Source: CAD feature listing. Evaluate the final solid. Frame: model axes, mm. A direction names the side the tool comes from. Give positions to 0.01 mm unless a question says otherwise; leave off trailing zeros. Write each loop counter-clockwise with the first axis right and the second up, starting at its lowest first coordinate (ties: lowest second). Pieces come first, ordered by that corner, then holes. Notation, with made-up numbers: (1, 37.25) -> (23, 37.25) arc R14 cw to (23, 58.25) -> close; hole circle Ø3 at (33, 89.5). An arc over 180 degrees is marked (long way). Answer as a JSON object with one key per item and string values. Group by question number.
Item 1: Section query B-B on x = 7. Return the cut outline in (y, z), plus the area to 3 significant figures.
Item 2: Section query A-A on z = 72.5. Return the cut outline in (x, y).
Item 3: First-contact query: pin 1 Ø6.5 at (x, z) = (-19.05, -31.75) entering from -Y; pin 2 Ø4 at (y, z) = (0, -241.3) entering from -X. Flat tips, straight axial feed; report the tip coordinate or a pass-through.
Item 4: Access query for faces 5 (the face through (0, -11.112, 4)), 6 (the face through (0, 12.7, 4)). Directions: +Z, -Z, +X, -X, +Y, -Y. A direction counts if a zero-diameter tool reaches every point of the face in a straight line with its end or side. Return the directions, or none.
Item 5: Pull-direction query (X, two-part tool) for faces 1 (the face through (-23.812, 0, 4)), 2 (the face through (-25.4, 0, 4)), 3 (the face through (0, -12.7, 4)), 4 (the face through (25.4, 0, 4)); classes: pulls with the +X half, pulls with the -X half, needs draft (parallel to the pull), parting line crosses it, or undercut.
Item 6: Ray query, probe 1 along X at (y, z) = (12.35, -31.75); probe 2 along Z at (x, y) = (-19.05, 11.5); probe 3 along X at (y, z) = (-5, 212.5). Return the intervals inside material, ascending. Write a range as from..to.
from build123d import *

# Parameters (mm, degrees)
SKETCH1_W               = 50.8
SKETCH1_H               = 25.4
BOSS_EXTRUDE1_DEPTH     = 279.4
SHELL1_T                = -1.5875
CUT_EXTRUDE1_DEPTH      = 281.839473721
CUT_EXTRUDE1_DEPTH_BACK = 281.839473721
SKETCH3_R               = 2.4892
CUT_EXTRUDE2_DEPTH      = 281.839473721
CUT_EXTRUDE2_DEPTH_BACK = 281.839473721
SKETCH4_R               = 2.4892


with BuildPart() as part:
    # Sketch1 → Boss-Extrude1 (new, symmetric)
    with BuildSketch(Plane.XY):
        Rectangle(SKETCH1_W, SKETCH1_H)
    extrude(amount=BOSS_EXTRUDE1_DEPTH, both=True)

    # Shell1
    shell1_openings = [part.faces().sort_by_distance(p)[0] for p in [
        (0, 0, 279.4),
        (0, 0, -279.4),
    ]]
    offset(amount=SHELL1_T, openings=shell1_openings, kind=Kind.INTERSECTION)

    # Sketch3 → Cut-Extrude1 (cut, two sides: drawn at the far end of the back side and taken through both)
    with BuildSketch(Plane(origin=(0, 0, 0), x_dir=(0, 0, -1), z_dir=(1, 0, 0)).offset(-CUT_EXTRUDE1_DEPTH_BACK)):
        with Locations((-266.7, 0)):
            Circle(SKETCH3_R)
        with Locations((-241.3, 0)):
            Circle(SKETCH3_R)
        with Locations((-215.9, 0)):
            Circle(SKETCH3_R)
        with Locations((215.9, 0)):
            Circle(SKETCH3_R)
        with Locations((241.3, 0)):
            Circle(SKETCH3_R)
        with Locations((266.7, 0)):
            Circle(SKETCH3_R)
    extrude(amount=CUT_EXTRUDE1_DEPTH + CUT_EXTRUDE1_DEPTH_BACK, mode=Mode.SUBTRACT)

    # Sketch4 → Cut-Extrude2 (cut, two sides: drawn at the far end of the back side and taken through both)
    with BuildSketch(Plane(origin=(0, 0, 0), x_dir=(1, 0, 0), z_dir=(0, 1, 0)).offset(-CUT_EXTRUDE2_DEPTH_BACK)):
        with Locations(Location((0, -31.75, 0), (0, 0, 270))):
            Circle(SKETCH4_R)
        with Locations(Location((-19.05, -31.75, 0), (0, 0, 270))):
            Circle(SKETCH4_R)
        with Locations(Location((0, 31.75, 0), (0, 0, 270))):
            Circle(SKETCH4_R)
        with Locations(Location((-19.05, 31.75, 0), (0, 0, 270))):
            Circle(SKETCH4_R)
    extrude(amount=CUT_EXTRUDE2_DEPTH + CUT_EXTRUDE2_DEPTH_BACK, mode=Mode.SUBTRACT)


solid = part.part
Worked answers:
{
 "1": {"outline": "(-12.7, -279.4) -> (-11.11, -279.4) -> (-11.11, 279.4) -> (-12.7, 279.4) -> close; (11.11, -279.4) -> (12.7, -279.4) -> (12.7, 279.4) -> (11.11, 279.4) -> close", "area": "1,770 mm^2"},
 "2": {"outline": "(-25.4, -12.7) -> (25.4, -12.7) -> (25.4, 12.7) -> (-25.4, 12.7) -> close; hole (-23.81, -11.11) -> (23.81, -11.11) -> (23.81, 11.11) -> (-23.81, 11.11) -> close"},
 "3": {"pin 1": "y = -12.7", "pin 2": "through"},
 "4": {"face 5": "+Z, -Z", "face 6": "+Z, -Z, +X, -X, +Y"},
 "5": {"face 1": "undercut", "face 2": "pulls with the -X half", "face 3": "needs draft", "face 4": "pulls with the +X half"},
 "6": {"probe 1": "-25.4..-21.54, -16.56..-2.49, 2.49..25.4", "probe 2": "-279.4..-34.24, -29.26..29.26, 34.24..279.4", "probe 3": "-25.4..-23.81, 23.81..25.4"}
}
